Autodesk Fusion 360 part; units mm, degrees
sketch "Boceto1" plane through (0, 0, 0) normal (1, 0, 0) x (0, 1, 0)
  line L0 (0, 0) -> (-15, 0)
  line L1 (0, 0) -> (0, 15)
  arc A0 (-15, 0) -> (0, 15) centre (-26.7699, 26.7699) ccw
  dimension "d1" = 15
  dimension "d2" = 15
extrude "Extruir1" add sketch "Boceto1" along normal blind 60
sketch "Boceto2" plane through (0, 0, 0) normal (0, 1, 0) x (-1, 0, 0)
  line L0 (0, 0) -> (0, 15)
  line L1 (0, 15) -> (-60, 15)
  line L2 (-60, 15) -> (-60, 0)
  line L3 (-60, 0) -> (0, 0)
  circle A0 centre (-45, 10) radius 1.5
  circle A1 centre (-15, 10) radius 1.5
  dimension "d7" = 3
  dimension "d10" = 3
extrude "Extruir2" cut sketch "Boceto2" against normal blind 4 contours A0 | A1
sketch "Boceto3" plane through (0, 0, 0) normal (0, 0, -1) x (1, 0, 0)
  line L0 (0, 15) -> (0, 0)
  line L1 (0, 0) -> (60, 0)
  line L2 (60, 0) -> (60, 15)
  line L3 (60, 15) -> (0, 15)
  circle A0 centre (10, 8) radius 1.5
  circle A1 centre (50, 8) radius 1.5
  dimension "d17" = 3
  dimension "d18" = 3
extrude "Extruir3" cut sketch "Boceto3" against normal blind 6 contours A0 | A1
Geometry: final body of the model. Coordinates: model frame, mm. Round coordinates to 2 decimals unless told otherwise and drop trailing zeros. Order: outer loops, then holes, each group sorted by start corner. A loop starts at its lowest first (then second) coordinate and runs counter-clockwise, first axis right, second up. Notation, with made-up numbers: (40.25, 21.25) -> (86.25, 21.25) arc R26 ccw to (86.25, 43.25) -> close; hole circle Ø5 at (-4.5, -31). An arc over 180 degrees is marked (long way). Use one line per item in the form item = value. Start each with the question number.
1. Line query: probe 1 along X at (y, z) = (-2.75, 10); probe 2 along Y at (x, z) = (10, 4.55); probe 3 along Y at (x, z) = (50, 1.8). Output: solid intervals per line, ascending.
2. Draft query along Y for faces 1 (the face through (49.675, -6.536, 2.174)), 2 (the face through (29.58, -5.985, 6.2)), 3 (the face through (45.325, -1.503, 8.536)). Return one class per face: pulls with the +Y half, pulls with the -Y half, needs draft (parallel to the pull), parting line crosses it, or undercut.
3. Pin query (flat end, axial travel): pin 1 Ø5 at (x, y) = (46.5, -5) entering from -Z; pin 2 Ø1.8 at (x, y) = (10, -8) entering from +Z; pin 3 Ø3.5 at (x, y) = (50, -8) entering from +Z; pin 4 Ø1 at (x, y) = (36.5, -5) entering from +Z. Return the tip coordinate at first contact, or that it passes through.
4. Cut plane A-A (y = -8). Return the cut outline in (x, z), then the cut area to 3 significant figures.
5. Cut plane C-C (z = 10). Return the cut outline in (x, y), then the cut area to 3 significant figures.
6. Cut plane D-D (y = -1.5). Return the cut outline in (x, z).
7. Cut plane B-B (x = 45). Return the cut outline in (y, z), then the cut area to 3 significant figures.
Solution:
q1.probe_1 = 0 to 13.5, 16.5 to 43.5, 46.5 to 60
q1.probe_2 = -6.5 to 0
q1.probe_3 = -11.55 to -9.5, -6.5 to 0
q2.face_1 = undercut
q2.face_2 = pulls with the -Y half
q2.face_3 = needs draft
q3.pin_1 = 0
q3.pin_2 = through
q3.pin_3 = 5.94
q3.pin_4 = 7.82
q4.outline = (0, 0) -> (8.5, 0) -> (8.5, 4.35) -> (0, 4.35) -> close; (11.5, 0) -> (48.5, 0) -> (48.5, 4.35) -> (11.5, 4.35) -> close; (51.5, 0) -> (60, 0) -> (60, 4.35) -> (51.5, 4.35) -> close
q4.area = 235 mm^2
q5.outline = (0, -2.81) -> (13.5, -2.81) -> (13.5, 0) -> (0, 0) -> close; (16.5, -2.81) -> (43.5, -2.81) -> (43.5, 0) -> (16.5, 0) -> close; (46.5, -2.81) -> (60, -2.81) -> (60, 0) -> (46.5, 0) -> close
q5.area = 152 mm^2
q6.outline = (0, 0) -> (60, 0) -> (60, 12.05) -> (0, 12.05) -> close; hole circle Ø3 at (15, 10); hole circle Ø3 at (45, 10)
q7.outline = (-15, 0) -> (0, 0) -> (0, 8.5) -> (-3.94, 8.5) arc R29.24 cw to start; (-1.83, 11.5) -> (0, 11.5) -> (0, 15) arc R29.24 cw to start
q7.area = 75.6 mm^2
